Verification items for the finished model (mm, model axes). A direction names the side the tool comes from. Round coordinates to 2 decimals unless told otherwise and drop trailing zeros. Write each loop counter-clockwise with the first axis right and the second up, starting at its lowest first coordinate (ties: lowest second). Pieces come first, ordered by that corner, then holes. Notation, with made-up numbers: M -35.5,43 L -15.5,43 A25 cw -15.5,61 Z; hole C 29,-30.5 d11. An arc over 180 degrees is marked long. Write each question's results on one line, items separated by ' | '.
from build123d import *

# Parameters (mm, degrees)
F0_R     = 9
F0_R_2   = 5.5
F1_DEPTH = 2.5
F0_R_3   = 3.175
F2_DEPTH = 3.5
F3_DEPTH = 5.8
F4_R     = 1.5


with BuildPart() as f1:
    # F0 (on Top) → F1 (new body)
    with BuildSketch(Plane.XY):
        Circle(F0_R)
        Circle(F0_R_2, mode=Mode.SUBTRACT)
    extrude(amount=F1_DEPTH)

    # F0 (on Top) → F2 (join, through all)
    with BuildSketch(Plane.XY):
        Circle(F0_R_2)
        Circle(F0_R_3, mode=Mode.SUBTRACT)
    extrude(amount=F2_DEPTH)

    # F0 (on Top) → F3 (join, through all)
    with BuildSketch(Plane.XY):
        Circle(F0_R_3)
    extrude(amount=F3_DEPTH)

    # F4
    f4_edges = [f1.edges().sort_by_distance(p)[0] for p in [
        (-9, 0, 0),
    ]]
    fillet(f4_edges, radius=F4_R)


solid = f1.part
1) Sectioned sample at C-C, the plane z = 3.8. Record the cut outline in (x, y) (3 decimals).
Calculated:
outline: C 0,0 d6.35
2) Depth check by flat-ended pin: P1, Ø3, axis at x = 4.5, z = 1.5, coming from the +Y side; P2, Ø3, axis at x = 0.5, z = 2, coming from the +Y side; P3, Ø1.5, axis at x = 0, z = 4, coming from the -Y side; P4, Ø1.5, axis at x = -7, z = 1.5, coming from the -Y side. Enter the tip coordinate at first touch or a pass-through.
Calculated:
P1: stops at y = 8.49 | P2: stops at y = 9 | P3: stops at y = -5.5 | P4: stops at y = -6.48
3) Material ranges on line 1 (Z direction, x = -1.25, y = -3.25); line 2 (Z direction, x = -5, y = -2.75); line 3 (X direction, y = 4.5, z = 1.35), recorded low to high. Write a range as [from, to].
Calculated:
line 1: z = [0, 3.5] | line 2: z = [0, 2.5] | line 3: x = [-7.79, 7.79]
4) Sectioned sample at D-D, the plane z = 2.75. Record the cut outline in (x, y), and give its area (3 significant figures).
Calculated:
outline: C 0,0 d11 | area: 95.0 mm²
5) Access from +Z, -Z, +X, -X, +Y, -Y to the whole of each face (thin tool, end or side, straight path). Record for faces 1 (the cylindrical face through (-1.19, -5.37, 2.99)), 2 (the cylindrical face through (-1.172, 8.923, 1.993)).
Calculated:
face 1: +Z | face 2: +Z, -Z
6) Sectioned sample at A-A, the plane x = 0. Record the cut outline in (y, z) (3 decimals), and give its area (3 significant figures).
Calculated:
outline: M -9,1.5 A1.5 ccw -7.5,0 L 7.5,0 A1.5 ccw 9,1.5 L 9,2.5 L 5.5,2.5 L 5.5,3.5 L 3.175,3.5 L 3.175,5.8 L -3.175,5.8 L -3.175,3.5 L -5.5,3.5 L -5.5,2.5 L -9,2.5 Z | area: 69.6 mm²
